Source: CAD feature listing. Evaluate the final solid. Frame: model axes, mm. Face numbers are marked on the shaded views. A direction names the side the tool comes from. Round coordinates to 2 decimals unless told otherwise and drop trailing zeros. Order: outer loops, then holes, each group sorted by start corner. A loop starts at its lowest first (then second) coordinate and runs counter-clockwise, first axis right, second up. Notation, with made-up numbers: (-21.5, -8.75) -> (-10.5, -8.75) arc R32 ccw to (-10.5, 23.25) -> close; hole circle Ø7 at (36, -29). An arc over 180 degrees is marked (long way). One line per item, written item: value. Start each with the question number.
1) Ray query, L1, parallel to Z at x = 17.5, y = 8; L2, parallel to X at y = 4.5, z = 16; L3, parallel to Z at x = 26.5, y = 0.75. Return the intervals inside material, ascending.
2) Reachability of the marked faces 1, 2, 3, 4 and 5 from +Z, -Z, +X, -X, +Y, -Y: full face, straight path, thin tool, end or side. Return the list, or none.
3) Section A-A (z = 45.5). Return the cut outline in (x, y), and give its area (3 significant figures).
4) Pin query (flat end, axial travel): P1, Ø2.5, axis at x = 17.5, z = 16.05, coming from the -Y side; P2, Ø5, axis at x = 4, z = 45.5, coming from the -Y side; P3, Ø2.5, axis at x = 43.5, y = 1.5, coming from the +Z side; P4, Ø10, axis at x = -4, z = 2.5, coming from the +Y side. Return the tip coordinate at first contact, or that it passes through.
5) Section B-B (x = 47.5). Return the cut outline in (y, z).
6) Section C-C (x = 17.5). Return the cut outline in (y, z).
7) Section D-D (z = 20). Return the cut outline in (x, y), and give its area (4 significant figures).
```python
from build123d import *

# Parameters (mm, degrees)
F0_R     = 1.45
F0_R_2   = 1.85
F0_R_3   = 1.5
F1_DEPTH = 3
F2_DEPTH = 13
F3_D     = 6
F3_DEPTH = 3
F3_TIP   = 1.8025818571


with BuildPart() as f1:
    # F0 (on Front) → F1 (new body)
    with BuildSketch(Plane.XZ):
        Polygon((-10.5, -5), (51.5, -5), (51.5, 12.5), (21.5, 12.5), (21.5, 12.0468574613), (13.5, 12.0468574613), (13.5, 35.0468574613), (8, 35.0468574613), (8, 49.5), (0, 49.5), (0, 3), (-10.5, 3), align=None)
        with Locations((-6.5, -1)):
            Circle(F0_R, mode=Mode.SUBTRACT)
        with Locations((26.5, -1)):
            Circle(F0_R, mode=Mode.SUBTRACT)
        with Locations((47.5, 8.5)):
            Circle(F0_R_2, mode=Mode.SUBTRACT)
        with Locations((4, 45.5)):
            Circle(F0_R_2, mode=Mode.SUBTRACT)
        Polygon((21.5, 12.0468574613), (21.5, 12.5), (21.5, 35.0468574613), (13.5, 35.0468574613), (13.5, 12.0468574613), align=None)
        with Locations((17.5, 16.0468574613)):
            Circle(F0_R_3, mode=Mode.SUBTRACT)
        with Locations((17.5, 31.0468574613)):
            Circle(F0_R_3, mode=Mode.SUBTRACT)
    extrude(amount=-F1_DEPTH)

    # F0 (on Front) → F2 (join)
    with BuildSketch(Plane.XZ):
        Polygon((21.5, 12.0468574613), (21.5, 12.5), (21.5, 35.0468574613), (13.5, 35.0468574613), (13.5, 12.0468574613), align=None)
        with Locations((17.5, 16.0468574613)):
            Circle(F0_R_3, mode=Mode.SUBTRACT)
        with Locations((17.5, 31.0468574613)):
            Circle(F0_R_3, mode=Mode.SUBTRACT)
    extrude(amount=-F2_DEPTH)

    # F3
    with Locations(Plane.XZ):
        with Locations((17.5, 31.0468574613), (17.5, 16.0468574613)):
            Hole(F3_D / 2, depth=F3_DEPTH)
            with Locations((0, 0, -(F3_DEPTH + F3_TIP / 2))):  # 118° drill point
                Cone(0, F3_D / 2, F3_TIP, mode=Mode.SUBTRACT)


solid = f1.part
```
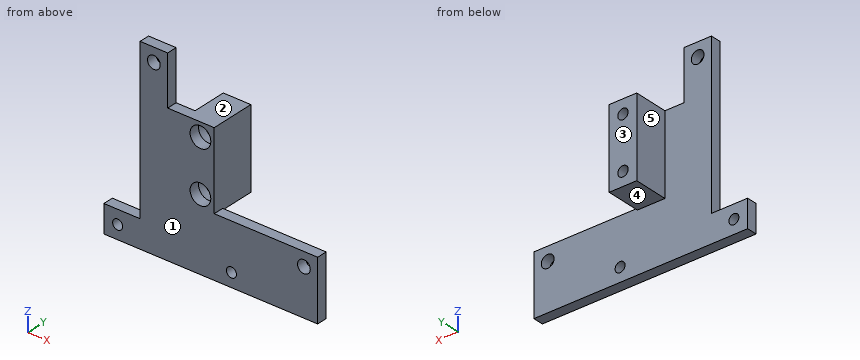
Findings:
1. L1: 12.05 to 14.55, 17.55 to 29.55, 32.55 to 35.05
1. L2: 13.5 to 16, 19 to 21.5
1. L3: -5 to -2.45, 0.45 to 12.5
2. face 1: +Z, -Z, +X, -X, -Y
2. face 2: +Z, +X, +Y, -Y
2. face 3: +Z, -Z, +X, -X, +Y
2. face 4: -Z, +X, -X, +Y
2. face 5: +Z, -Z, -X, +Y
3. outline: (0, 0) -> (2.15, 0) -> (2.15, 3) -> (0, 3) -> close; (5.85, 0) -> (8, 0) -> (8, 3) -> (5.85, 3) -> close
3. area: 12.9 mm2
4. P1: through
4. P2: y = 0
4. P3: z = 12.5
4. P4: y = 3
5. outline: (0, -5) -> (3, -5) -> (3, 6.65) -> (0, 6.65) -> close; (0, 10.35) -> (3, 10.35) -> (3, 12.5) -> (0, 12.5) -> close
6. outline: (0, -5) -> (3, -5) -> (3, 12.05) -> (13, 12.05) -> (13, 14.55) -> (3.9, 14.55) -> (3, 13.05) -> (0, 13.05) -> close; (0, 19.05) -> (3, 19.05) -> (3.9, 17.55) -> (13, 17.55) -> (13, 29.55) -> (3.9, 29.55) -> (3, 28.05) -> (0, 28.05) -> close; (0, 34.05) -> (3, 34.05) -> (3.9, 32.55) -> (13, 32.55) -> (13, 35.05) -> (0, 35.05) -> close
7. outline: (0, 0) -> (21.5, 0) -> (21.5, 13) -> (13.5, 13) -> (13.5, 3) -> (0, 3) -> close
7. area: 144.5 mm2
